Could you check a few things on this model? Use its own coordinates, in mm. A direction names the side the tool comes from. Round coordinates to 2 decimals unless told otherwise and drop trailing zeros. Loops run counter-clockwise (first coordinate to the right, second up) from the corner with the lowest first, then second, coordinate; pieces in that order, holes last. Notation, with made-up numbers: (-20.75, 47.25) -> (32.25, 47.25) arc R17 ccw to (32.25, 60.25) -> close; hole circle Ø1 at (25.5, 84.5). An arc over 180 degrees is marked (long way). One line per item, written item: value.
from build123d import *

# Parameters (mm, degrees)
F3_SIZE = 0.5


with BuildPart() as f1:
    # F0 (on Front) → F1 (revolve)
    with BuildSketch(Plane.XZ):
        Polygon((5, 3.5), (4, 3.5), (4, 0), (11, 0), (11, 3.5), (9, 3.5), (9, 3), (5, 3), align=None)
    revolve(axis=Axis((0, 0, 3.124244744), (0, 0, 1)))

    # F2: F1 across plane


with BuildPart() as f1_1:
    add(f1.part)
    add(f1.part.mirror(Plane.XY))

    # F3
    f3_edges = [f1_1.edges().sort_by_distance(p)[0] for p in [
        (-11, 0, 3.5),
        (-11, 0, -3.5),
        (-4, 0, 3.5),
        (-4, 0, -3.5),
    ]]
    chamfer(f3_edges, length=F3_SIZE)


solid = f1_1.part
(1) Thinking about a two-plate mould opening in X: for faces 1 (the face through (8, 5, -3.5)), 2 (the face through (4, -4, 3)), 3 (the face through (-1.172, 8.923, 3.246)), which applies, released by +X, released by -X, zero draft, split by the parting line, or undercut?
Recorded:
face 1: zero draft
face 2: undercut
face 3: undercut
(2) I'm going to push flat-ended pins straight in: pin 1 Ø1 at (x, z) = (5, -1.5) entering from -Y; pin 2 Ø2 at (y, z) = (-2, 0) entering from +X; pin 3 Ø2 at (x, z) = (-3.5, -2.5) entering from -Y. Where does each tip first touch, or does it pass through?
Recorded:
pin 1: y = -10.04
pin 2: x = 10.95
pin 3: y = -10.71
(3) For faces 4 (the face through (-1.08, -4.88, -3.25)), 5 (the face through (-1.08, -4.88, 3.25)), 6 (the face through (8, 5, 3.5)), which set-ups out of +Z, -Z, +X, -X, +Y, -Y let a thin tool reach every point of the face, with its end or its side?
Recorded:
face 4: -Z
face 5: +Z
face 6: +Z, +X, -X, +Y, -Y
(4) If I drill on L1, parallel to Y at x = 0, z = 3.3; L2, parallel to Y at x = 0, z = 1.8; L3, parallel to Y at x = 0, z = -3.2, over which ranges is the centre line in solid material (lowest first)?
Recorded:
L1: -10.7 to -9, -5 to -4.3, 4.3 to 5, 9 to 10.7
L2: -11 to -4, 4 to 11
L3: -10.8 to -9, -5 to -4.2, 4.2 to 5, 9 to 10.8
(5) If we section it at C-C, the plane z = -2.25: Please give me the cut outline in (x, y), then the cut area to 3 significant figures.
Recorded:
outline: circle Ø22 at (0, 0); hole circle Ø8 at (0, 0)
area: 330 mm²
